```python
from build123d import *

# Parameters (mm, degrees)
F0_W     = 41
F0_H     = 2.1
F1_DEPTH = 6
F2_W     = 16.4
F2_H     = 3
F3_DEPTH = 4
F4_W     = 43.9
F4_H     = 6.6
F5_DEPTH = 1


with BuildPart() as f1:
    # F0 (on Top) → F1 (new body)
    with BuildSketch(Plane.XY):
        with BuildLine():
            ThreePointArc((3, 2.569533), (0, -3.95), (-3, 2.569533))
            ThreePointArc((-3, 2.569533), (-3.084459, 3.66229), (-4.177215, 3.577831))
            ThreePointArc((-4.177215, 3.577831), (-5.395403, -1.06753), (-2.5, -4.898979))
            Line((-2.5, -4.898979), (-2.5, -6.45))
            Line((-2.5, -6.45), (-14.5, -6.45))
            Line((-14.5, -6.45), (-14.5, -13.05))
            Line((-14.5, -13.05), (29.4, -13.05))
            Line((29.4, -13.05), (29.4, -6.45))
            Line((29.4, -6.45), (2.5, -6.45))
            Line((2.5, -6.45), (2.5, -4.898979))
            ThreePointArc((2.5, -4.898979), (5.395403, -1.06753), (4.177215, 3.577831))
            ThreePointArc((4.177215, 3.577831), (3.084459, 3.66229), (3, 2.569533))
        make_face()
        with Locations((7.5, -10.5)):
            Rectangle(F0_W, F0_H, mode=Mode.SUBTRACT)
    extrude(amount=F1_DEPTH)

    # F2 (on face) → F3 (cut)
    with BuildSketch(Plane.XY.offset(6)):
        with Locations((21.2, -7.95)):
            Rectangle(F2_W, F2_H)
    extrude(amount=-F3_DEPTH, mode=Mode.SUBTRACT)

    # F4 (on face) → F5 (join)
    with BuildSketch(Plane(origin=(0, 0, 0), x_dir=(1, 0, 0), z_dir=(0, 0, -1))):
        with Locations((7.45, 9.75)):
            Rectangle(F4_W, F4_H)
    extrude(amount=-F5_DEPTH)


solid = f1.part
```
The model under review builds one solid part; all positions refer to its coordinate system, in mm. A direction names the side the tool comes from. Round coordinates to 2 decimals unless told otherwise and drop trailing zeros. Write each loop counter-clockwise with the first axis right and the second up, starting at its lowest first coordinate (ties: lowest second). Pieces come first, ordered by that corner, then holes.
(1) We need section A-A on y = 0. Give the boundary of the cut face in (x, z).
(2) Machinability: for faces 1 (the flat face through (7, -11, 1)), 2 (the flat face through (21, -8, 2)), 3 (the flat face through (-8, -6.45, 3)), which of the approach directions +Z, -Z, +X, -X, +Y, -Y give a long, thin tool a straight path to every point of the face, cutting with its end or side? Answer none if there is none.
(3) We need section B-B on x = -5. Give the boundary of the cut face in (y, z).
(4) We need section D-D on x = 0. Give the boundary of the cut face in (y, z).
(5) Mouldability with a two-part tool opening along Y and no side actions: class faces 4 (the flat face through (2, -8, 6)), 5 (the flat face through (7, -13.05, 3)), 6 (the flat face through (2.5, -6, 3)) as +Y half, -Y half, draft (parallel to the pull), parting line (faces both ways), or undercut.
(6) We need section C-C on z = 4.7. Give the boundary of the cut face in (x, y) (3 decimals).
(7) Insertion check: pin 1 (0.5 mm diameter, centred on y = -5.5, z = 2, fed in from -X); pin 2 (1.5 mm diameter, centred on x = 28.5, z = 4, fed in from +Y); pin 3 (1.8 mm diameter, centred on x = 9.5, z = 4, fed in from +Y); pin 4 (1 mm diameter, centred on x = 2.5, y = 0.5, fed in from -Z). Each pin has a flat end and moves straight along its axis. Give the tip position at first contact, or say it passes through.
(8) Wall thickness on L1, parallel to Y at x = 9, z = 3.9; L2, parallel to X at y = 0, z = 4; L3, parallel to X at y = -10, z = 5: over which ranges is each line inside the solid? List them lowest first.
Findings below:
1. outline: (-5.5, 0) - (-3.95, 0) - (-3.95, 6) - (-5.5, 6) - close; (3.95, 0) - (5.5, 0) - (5.5, 6) - (3.95, 6) - close
2. face 1: +Z
2. face 2: +Z, +X, +Y
2. face 3: +Z, -Z, -X
3. outline: (-13.05, 0) - (-6.45, 0) - (-6.45, 6) - (-9.45, 6) - (-9.45, 1) - (-11.55, 1) - (-11.55, 6) - (-13.05, 6) - close; (-2.29, 0) - (2.29, 0) - (2.29, 6) - (-2.29, 6) - close
4. outline: (-13.05, 0) - (-3.95, 0) - (-3.95, 6) - (-9.45, 6) - (-9.45, 1) - (-11.55, 1) - (-11.55, 6) - (-13.05, 6) - close
5. face 4: draft
5. face 5: -Y half
5. face 6: undercut
6. outline: (-14.5, -13.05) - (29.4, -13.05) - (29.4, -9.45) - (28, -9.45) - (28, -11.55) - (-13, -11.55) - (-13, -9.45) - (13, -9.45) - (13, -6.45) - (2.5, -6.45) - (2.5, -4.899) arc R5.5 ccw to (4.177, 3.578) arc R0.775 ccw to (3, 2.57) arc R3.95 cw (long way) to (-3, 2.57) arc R0.775 ccw to (-4.177, 3.578) arc R5.5 ccw to (-2.5, -4.899) - (-2.5, -6.45) - (-14.5, -6.45) - close
7. pin 1: stops at x = -2.5
7. pin 2: stops at y = -9.45
7. pin 3: stops at y = -6.45
7. pin 4: passes through
8. L1: y = -13.05 to -11.55, -9.45 to -6.45
8. L2: x = -5.5 to -3.95, 3.95 to 5.5
8. L3: x = -14.5 to -13, 28 to 29.4
